from build123d import *

# Parameters (mm, degrees)
F2_R = 25.4
F3_R = 50.8


with BuildPart() as f1:
    # F0 (on Front) → F1 (revolve)
    with BuildSketch(Plane.XZ):
        with BuildLine():
            Line((-152.4, 0), (0, 0))
            Line((0, 0), (0, 294.64))
            ThreePointArc((0, 294.64), (-70.59093, 277.01008), (-127, 231.054554))
            Line((-127, 231.054554), (-152.4, 0))
        make_face()
    revolve(axis=Axis((0, 0, 147.32), (0, 0, -1)))

    # F2
    f2_edges = [f1.edges().sort_by_distance(p)[0] for p in [
        (152.4, 0, 0),
    ]]
    fillet(f2_edges, radius=F2_R)

    # F3
    f3_edges = [f1.edges().sort_by_distance(p)[0] for p in [
        (127, 0, 231.054554),
    ]]
    fillet(f3_edges, radius=F3_R)


solid = f1.part
For this review, take the finished solid that the model builds, in its own axes (mm). Round coordinates to 2 decimals unless told otherwise and drop trailing zeros. Loops run counter-clockwise (first coordinate to the right, second up) from the corner with the lowest first, then second, coordinate; pieces in that order, holes last. Notation, with made-up numbers: (10, 57) - (29, 57) arc R23 ccw to (29, 87) - close; hole circle Ø2 at (-26, 64). An arc over 180 degrees is marked (long way). One line per item, written item: value. Start each with the question number.
Item 1: Clearance check with flat-ended pins moving along their axes: pin 1 Ø10 at (x, z) = (-15, 224.5) entering from +Y; pin 2 Ø8 at (x, z) = (-3, 202.5) entering from +Y; pin 3 Ø6 at (y, z) = (-98, 181) entering from -X. State where each tip first meets the part, or that it passes through.
Item 2: Take a section at A-A (z = 101). Give the boundary of the cut face in (x, y).
Item 3: For L1, parallel to Y at x = -12.5, z = 210; L2, parallel to Z at x = 7, y = -87; L3, parallel to Z at x = 55.5, y = 77, list the stretches that pass through material, from the lowest coordinate up.
Item 4: Take a section at B-B (z = 50). Give the boundary of the cut face in (x, y), plus the area to 3 significant figures.
Answer below:
1. pin 1: stops at y = 127.33
1. pin 2: stops at y = 130.55
1. pin 3: stops at x = -92.4
2. outline: circle Ø282.59 at (0, 0)
3. L1: y = -128.71 to 128.71
3. L2: z = 0 to 267.41
3. L3: z = 0 to 262.11
4. outline: circle Ø293.81 at (0, 0)
4. area: 67,800 mm2
